Part print with two shaded views. Sizes in mm from the minimum x, y, z corner. A direction names the side the tool comes from. Round coordinates to 2 decimals unless told otherwise and drop trailing zeros. Order: outer loops, then holes, each group sorted by start corner. A loop starts at its lowest first (then second) coordinate and runs counter-clockwise, first axis right, second up. Notation, with made-up numbers: M 55,80 L 80,80 A19 cw 80,96 Z; hole C 15,-30 d4. An arc over 180 degrees is marked long. One line per question, with ' | ' between items.
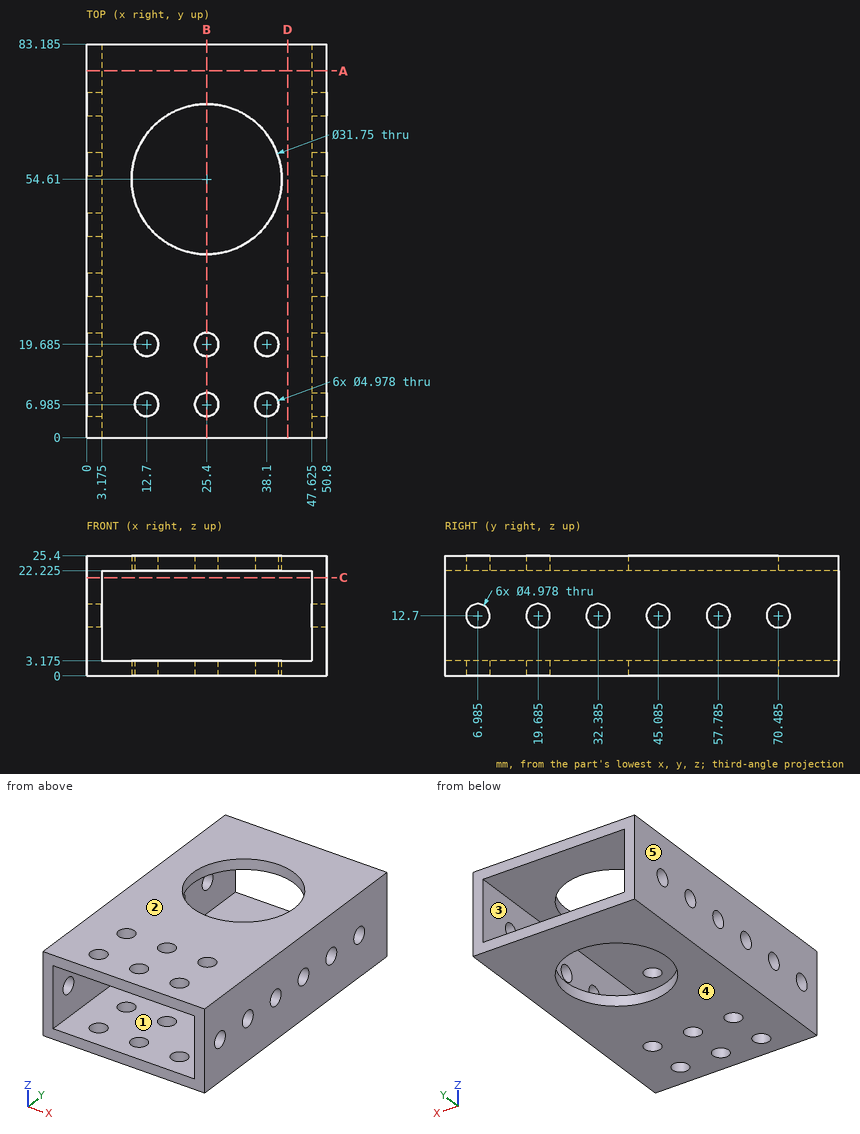
1) Saw through at A-A (y = 77.5). List the corners of the cut face in (x, z) (1 decimal).
The answers:
outline: M 0,0 L 50.8,0 L 50.8,25.4 L 0,25.4 Z; hole M 3.2,3.2 L 47.6,3.2 L 47.6,22.2 L 3.2,22.2 Z
2) Which spindle directions (+Z, -Z, +X, -X, +Y, -Y) get a long thin tool onto all of the face, cutting with end or side? Do the marked faces 1 and 2. Say none if no direction does.
The answers:
face 1: +Y, -Y | face 2: +Z, +X, -X, +Y, -Y
3) Saw through at C-C (z = 20.75). List the corners of the cut face in (x, y) (1 decimal).
The answers:
outline: M 0,0 L 3.2,0 L 3.2,83.2 L 0,83.2 Z; M 47.6,0 L 50.8,0 L 50.8,83.2 L 47.6,83.2 Z
4) Drop a flat-ended pin along its axis: pin 1 (4.5 mm diameter, centred on y = 70.485, z = 12.7, fed in from +X). Give the stop position or say it passes through.
The answers:
pin 1: passes through
5) Two-plate mould, pull along Z, no slides. Class the marked faces 3, 4 and 5: released by +Z, released by -Z, zero draft, split by the parting line, or undercut.
The answers:
face 3: undercut | face 4: released by -Z | face 5: zero draft
6) Saw through at B-B (x = 25.4). Give the number of separate pieces and of enclosed holes in the cut face.
The answers:
separate pieces: 8 | enclosed holes: 0
7) Probe line 1 (Z direction, x = 7.5, y = 43.5) (1 decimal); line 2 (X direction, y = 12, z = 15.75) (1 decimal); line 3 (Y direction, x = 12.7, z = 0.85) (1 decimal). List the from-to ranges inside material, lowest first. Write a range as [from, to].
The answers:
line 1: z = [0, 3.2], [22.2, 25.4] | line 2: x = [0, 3.2], [47.6, 50.8] | line 3: y = [0, 4.5], [9.5, 17.2], [22.2, 45.1], [64.1, 83.2]
8) Saw through at D-D (x = 42.5). List the corners of the cut face in (y, z) (1 decimal).
The answers:
outline: M 0,0 L 83.2,0 L 83.2,3.2 L 0,3.2 Z; M 0,22.2 L 83.2,22.2 L 83.2,25.4 L 0,25.4 Z
